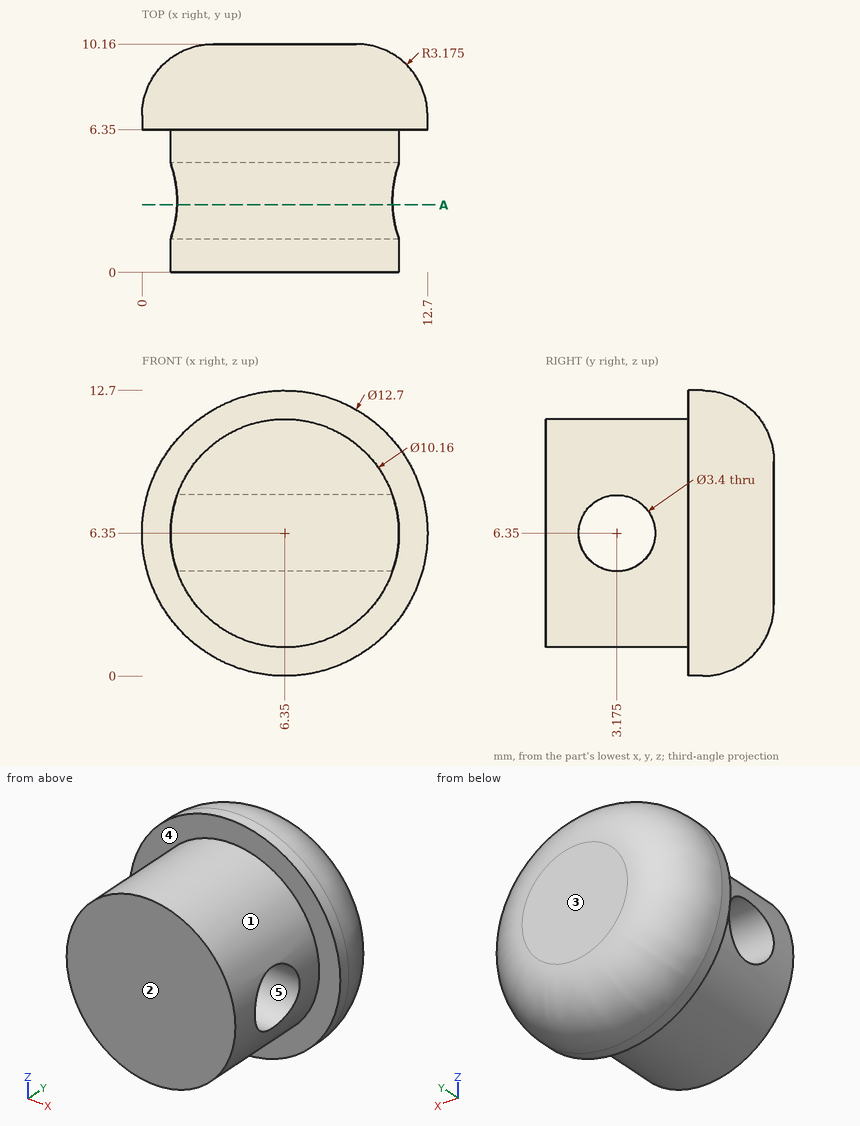
Input: dimensioned drawing with shaded views. Units: mm. Origin: part minimum x, y, z. A direction names the side the tool comes from. Give positions to 0.01 mm unless a question says otherwise; leave off trailing zeros. Loops run counter-clockwise (first coordinate to the right, second up) from the corner with the lowest first, then second, coordinate; pieces in that order, holes last. Notation, with made-up numbers: M 52,30 L 93,30 A19 cw 93,54 Z; hole C 65,30.25 d4. An arc over 180 degrees is marked long. Put each result on its own line as item: value.
1) Mould query, pull axis Y, two halves, no side actions, for the marked faces 3, 4 and 5. Classes: released by +Y, released by -Y, zero draft, split by the parting line, or undercut.
Computed values:
face 3: released by +Y
face 4: released by -Y
face 5: undercut
2) First-contact query: P1, Ø1, axis at x = 10, z = 7.5, coming from the +Y side; P2, Ø2, axis at y = 3.175, z = 6.35, coming from the -X side; P3, Ø4, axis at y = 5, z = 7, coming from the +X side; P4, Ø3, axis at y = 8, z = 3.5, coming from the -X side. Flat tips, straight axial feed; report the tip coordinate or a pass-through.
Computed values:
P1: stops at y = 10.16
P2: passes through
P3: stops at x = 12.7
P4: stops at x = 0.2
3) Material intervals for L1, parallel to Y at x = 8.5, z = 6.35 (3 decimals); L2, parallel to Z at x = 8.75, y = 3.5; L3, parallel to Z at x = 2, y = 2.25, sorted ascending. Write a range as from..to.
Computed values:
L1: y = 0..1.475, 4.875..10.16
L2: z = 1.87..4.68, 8.02..10.83
L3: z = 3.73..4.92, 7.78..8.97
4) Cut plane A-A, the plane y = 3. Return the cut outline in (x, z), plus the area to 3 significant figures.
Computed values:
outline: M 1.56,4.66 A5.08 ccw 11.14,4.66 Z; M 1.56,8.04 L 11.14,8.04 A5.08 ccw Z
area: 47.4 mm^2
5) Reachability of the marked faces 1 and 2 from +Z, -Z, +X, -X, +Y, -Y: full face, straight path, thin tool, end or side. Return the list, or none.
Computed values:
face 1: -Y
face 2: +Z, -Z, +X, -X, -Y
